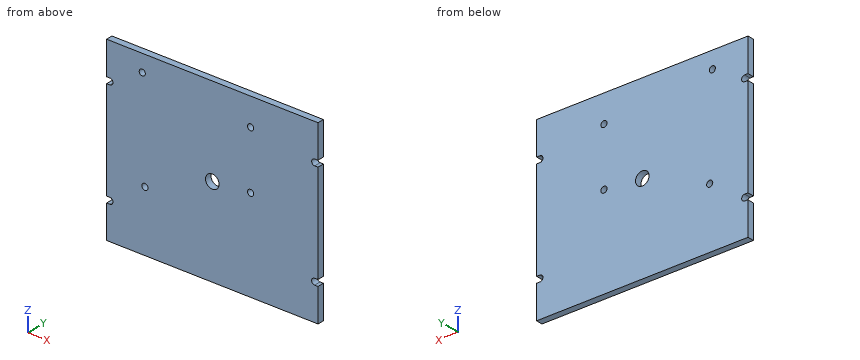
from build123d import *

# Parameters (mm, degrees)
SKETCH1_W               = 101.6
SKETCH1_H               = 85.725
BOSS_EXTRUDE1_DEPTH     = 3.175
F_4_CLEARANCE_HOLE1_D   = 2.9464
CUT_EXTRUDE1_DEPTH      = 67.542576831
F_1_4_CLEARANCE_HOLE1_D = 6.5278


with BuildPart() as part:
    # Sketch1 → Boss-Extrude1 (new body)
    with BuildSketch(Plane(origin=(0, 0, 0), x_dir=(1, 0, 0), z_dir=(0, 1, 0))):
        Rectangle(SKETCH1_W, SKETCH1_H)
    extrude(amount=BOSS_EXTRUDE1_DEPTH)

    # #4 Clearance Hole1 (through all)
    with Locations(Plane(origin=(0, 0, 0), x_dir=(-1, 0, 0), z_dir=(0, -1, 0))):
        with Locations((-18.415, -1.6525), (-18.415, -29.5925), (33.655, -34.6725), (32.385, 13.5875)):
            Hole(F_4_CLEARANCE_HOLE1_D / 2)

    # Sketch4 → Cut-Extrude1 (cut, through all)
    with BuildSketch(Plane.XZ):
        with BuildLine():
            Line((49.2125, -26.8732), (50.8, -26.8732))
            Line((50.8, -26.8732), (50.8, -23.9268))
            Line((50.8, -23.9268), (49.2125, -23.9268))
            ThreePointArc((49.2125, -23.9268), (47.7393, -25.4), (49.2125, -26.8732))
        make_face()
        with BuildLine():
            Line((49.2125, 26.8732), (50.8, 26.8732))
            Line((50.8, 26.8732), (50.8, 23.9268))
            Line((50.8, 23.9268), (49.2125, 23.9268))
            ThreePointArc((49.2125, 23.9268), (47.7393, 25.4), (49.2125, 26.8732))
        make_face()
        with BuildLine():
            Line((-49.2125, 26.8732), (-50.8, 26.8732))
            Line((-50.8, 26.8732), (-50.8, 23.9268))
            Line((-50.8, 23.9268), (-49.2125, 23.9268))
            ThreePointArc((-49.2125, 23.9268), (-47.7393, 25.4), (-49.2125, 26.8732))
        make_face()
        with BuildLine():
            Line((-49.2125, -23.9268), (-50.8, -23.9268))
            Line((-50.8, -23.9268), (-50.8, -26.8732))
            Line((-50.8, -26.8732), (-49.2125, -26.8732))
            ThreePointArc((-49.2125, -26.8732), (-47.7393, -25.4), (-49.2125, -23.9268))
        make_face()
    extrude(amount=-CUT_EXTRUDE1_DEPTH, mode=Mode.SUBTRACT)

    # 1/4 Clearance Hole1 (through all)
    with Locations(Plane(origin=(0, 0, 0), x_dir=(-1, 0, 0), z_dir=(0, -1, 0))):
        with Locations((0, 0)):
            Hole(F_1_4_CLEARANCE_HOLE1_D / 2)


solid = part.part
Read the model definition and answer for the solid it produces. Units are mm, in the model's axes. Round coordinates to 2 decimals unless told otherwise and drop trailing zeros. Loops run counter-clockwise (first coordinate to the right, second up) from the corner with the lowest first, then second, coordinate; pieces in that order, holes last.
Q1. Consider probe 1 along X at (y, z) = (0.85, -14.5); probe 2 along X at (y, z) = (1.6, 36); probe 3 along X at (y, z) = (0.9, 24.5). Determine where each line is inside the solid, lowest interval first.
Q2. Section A-A on x = 0 is taken. Write down the section's boundary in (y, z) (1 decimal), and give its area (3 significant figures).
Q3. Section B-B on z = 25.4 is taken. Write down the section's boundary in (x, y) (3 decimals).
Output:
1. probe 1: x = -50.8 to -33.54, -31.23 to 50.8
1. probe 2: x = -50.8 to -34.29, -33.02 to 50.8
1. probe 3: x = -48.05 to 48.05
2. outline: (0, -42.9) - (3.2, -42.9) - (3.2, -3.3) - (0, -3.3) - close; (0, 3.3) - (3.2, 3.3) - (3.2, 42.9) - (0, 42.9) - close
2. area: 251 mm2
3. outline: (-47.739, 0) - (47.739, 0) - (47.739, 3.175) - (-47.739, 3.175) - close
